Design review of the part built by this model. Coordinates are the model's own, in mm. A direction names the side the tool comes from. Coordinates: 2 decimals unless noted, no trailing zeros. Write each loop counter-clockwise with the first axis right and the second up, starting at its lowest first coordinate (ties: lowest second). Pieces come first, ordered by that corner, then holes. Notation, with made-up numbers: M -28,44.5 L 6,44.5 A24 cw 6,58.5 Z; hole C 78.25,-8 d8. An arc over 180 degrees is marked long. One line per question, with ' | ' between items.
from build123d import *

# Parameters (mm, degrees)
F0_R     = 6.35
F1_DEPTH = 23.1902
F3_DEPTH = 23.1912
F5_R     = 2.4765
F6_DEPTH = 3.81
F7_R     = 1.5875
F8_DEPTH = 1.5885001


with BuildPart() as f1:
    # F0 (on Right) → F1 (new body)
    with BuildSketch(Plane.YZ):
        Circle(F0_R)
    extrude(amount=F1_DEPTH)

    # F2 (on face) → F3 (cut, through all)
    with BuildSketch(Plane.YZ.offset(23.1902)):
        with BuildLine():
            Line((6.2781560788, 0.9525), (-6.2781560788, 0.9525))
            ThreePointArc((-6.2781560788, 0.9525), (0, -6.35), (6.2781560788, 0.9525))
        make_face()
    extrude(amount=-F3_DEPTH, mode=Mode.SUBTRACT)

    # F5 (on offset) → F6 (cut)
    with BuildSketch(Plane(origin=(0, 0, 6.35), x_dir=(1, 0, 0), z_dir=(0, 0, -1))):
        with Locations((4.69265, 0)):
            Circle(F5_R)
        with Locations((18.49755, 0)):
            Circle(F5_R)
    extrude(amount=F6_DEPTH, mode=Mode.SUBTRACT)

    # F7 (on face) → F8 (cut, through all)
    with BuildSketch(Plane.XY.offset(2.54)):
        with Locations((4.69265, 0)):
            Circle(F7_R)
        with Locations((18.49755, 0)):
            Circle(F7_R)
    extrude(amount=-F8_DEPTH, mode=Mode.SUBTRACT)


solid = f1.part
1. To check wall thickness, follow line 1 along X through (y, z) = (0, 5.35); line 2 along X through (y, z) = (-1.5, 6.05); line 3 along Z through (x, y) = (18.5, 2). State the ranges of each line that lie inside material, in increasing order. Write a range as [from, to].
Answer sheet:
line 1: [0, 2.22], [7.17, 16.02], [20.97, 23.19] | line 2: [0, 2.72], [6.66, 16.53], [20.47, 23.19] | line 3: [0.95, 2.54]
2. Draft analysis for pull direction X (two halves, no side actions). For faces 3 (the face through (0, 0, 3)), 4 (the face through (23.19, 0, 3)), 5 (the face through (5, 2, 2.54)), 6 (the face through (16.91, 0.07, 1.76)), state which applies: pulls with the +X half, pulls with the -X half, needs draft (parallel to the pull), parting line crosses it, or undercut.
Answer sheet:
face 3: pulls with the -X half | face 4: pulls with the +X half | face 5: undercut | face 6: undercut
3. Take a section at C-C (z = 5.05). Write out the cut boundary in (x, y).
Answer sheet:
outline: M 0,-3.85 L 23.19,-3.85 L 23.19,3.85 L 0,3.85 Z; hole C 4.69,0 d4.95; hole C 18.5,0 d4.95
4. Take a section at A-A (y = 0). Write out the cut boundary in (x, z), then the cut area to 3 significant figures.
Answer sheet:
outline: M 0,0.95 L 3.11,0.95 L 3.11,2.54 L 2.22,2.54 L 2.22,6.35 L 0,6.35 Z; M 6.28,0.95 L 16.91,0.95 L 16.91,2.54 L 16.02,2.54 L 16.02,6.35 L 7.17,6.35 L 7.17,2.54 L 6.28,2.54 Z; M 20.09,0.95 L 23.19,0.95 L 23.19,6.35 L 20.97,6.35 L 20.97,2.54 L 20.09,2.54 Z | area: 77.3 mm^2
5. Take a section at B-B (x = 18.25). Write out the cut boundary in (y, z).
Answer sheet:
outline: M -6.28,0.95 L -1.57,0.95 L -1.57,2.54 L -2.46,2.54 L -2.46,5.85 A6.35 ccw Z; M 1.57,0.95 L 6.28,0.95 A6.35 ccw 2.46,5.85 L 2.46,2.54 L 1.57,2.54 Z
6. Tool access review of faces 1 (the face through (5.835, 2.197, 4.472)), 2 (the face through (11.43, 0.13, 6.35)): name each direction out of +Z, -Z, +X, -X, +Y, -Y from which nothing blocks a thin tool from reaching the whole face with its end or side.
Answer sheet:
face 1: +Z | face 2: +Z, +X, -X
7. Insertion check: pin 1 Ø1.5 at (x, z) = (16, 5) entering from -Y; pin 2 Ø3.5 at (x, y) = (4.69, 0) entering from -Z; pin 3 Ø1.5 at (x, y) = (18.5, 1) entering from +Z; pin 4 Ø5 at (x, y) = (4, -2.5) entering from +Z. Each pin has a flat end and moves straight along its axis. Give the tip position at first contact, or say it passes through.
Answer sheet:
pin 1: y = -4.72 | pin 2: z = 0.95 | pin 3: z = 2.54 | pin 4: z = 6.32
8. Take a section at D-D (y = -2.75). Write out the cut boundary in (x, z), then the cut area to 3 significant figures.
Answer sheet:
outline: M 0,0.95 L 23.19,0.95 L 23.19,5.72 L 0,5.72 Z | area: 111 mm^2
